from build123d import *

# Parameters (mm, degrees)
EXTRUDE_THIN1_DEPTH     = 60
CUT_EXTRUDE1_DEPTH      = 83.492423895
CUT_EXTRUDE1_DEPTH_BACK = 83.492423895


with BuildPart() as part:
    # Sketch1 → Extrude-Thin1 (new, symmetric)
    with BuildSketch(Plane(origin=(0, 0, 0), x_dir=(1, 0, 0), z_dir=(0, 1, 0))):
        with BuildLine():
            Line((25, -23), (-25, -23))
            ThreePointArc((-25, -23), (-30.656854249, -20.656854249), (-33, -15))
            Line((-33, -15), (-33, 15))
            ThreePointArc((-33, 15), (-30.656854249, 20.656854249), (-25, 23))
            Line((-25, 23), (25, 23))
            ThreePointArc((25, 23), (30.656854249, 20.656854249), (33, 15))
            Line((33, 15), (33, -15))
            ThreePointArc((33, -15), (30.656854249, -20.656854249), (25, -23))
        make_face()
        with BuildLine():
            Line((25, -20), (-25, -20))
            ThreePointArc((-25, -20), (-28.535533906, -18.535533906), (-30, -15))
            Line((-30, -15), (-30, 15))
            ThreePointArc((-30, 15), (-28.535533906, 18.535533906), (-25, 20))
            Line((-25, 20), (25, 20))
            ThreePointArc((25, 20), (28.535533906, 18.535533906), (30, 15))
            Line((30, 15), (30, -15))
            ThreePointArc((30, -15), (28.535533906, -18.535533906), (25, -20))
        make_face(mode=Mode.SUBTRACT)
    extrude(amount=EXTRUDE_THIN1_DEPTH, both=True)

    # Sketch3 → Cut-Extrude1 (cut, two sides: drawn at the far end of the back side and taken through both)
    with BuildSketch(Plane(origin=(0, 0, -23), x_dir=(-1, 0, 0), z_dir=(0, 0, -1)).offset(-CUT_EXTRUDE1_DEPTH_BACK)):
        with BuildLine():
            Line((-5, -40.937612565), (-5, 39.062387435))
            ThreePointArc((-5, 39.062387435), (0, 44.062387435), (5, 39.062387435))
            Line((5, 39.062387435), (5, -40.937612565))
            ThreePointArc((5, -40.937612565), (0, -45.937612565), (-5, -40.937612565))
        make_face()
    extrude(amount=CUT_EXTRUDE1_DEPTH + CUT_EXTRUDE1_DEPTH_BACK, mode=Mode.SUBTRACT)


solid = part.part
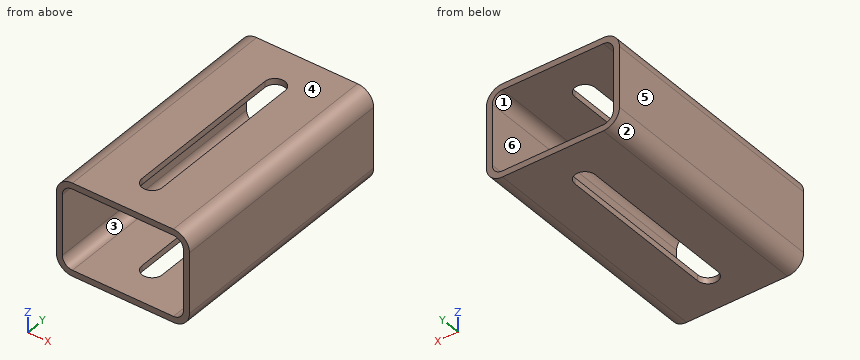
Check sheet for the modelled part. Datum: model origin and axes. Units: mm. Face numbers are marked on the shaded views. A direction names the side the tool comes from. Round coordinates to 2 decimals unless told otherwise and drop trailing zeros. Loops run counter-clockwise (first coordinate to the right, second up) from the corner with the lowest first, then second, coordinate; pieces in that order, holes last. Notation, with made-up numbers: M 71.25,-38.5 L 117.25,-38.5 A28 cw 117.25,-1.5 Z; hole C -19.75,-24 d2. An arc over 180 degrees is marked long. One line per item, written item: value.
(1) Access from +Z, -Z, +X, -X, +Y, -Y to the whole of each face (thin tool, end or side, straight path). Record for the marked faces 5 and 6.
Computed values:
face 5: +Z, -Z, -X, +Y, -Y
face 6: +Y, -Y
(2) Sectioned sample at D-D, the plane x = 0. Record the cut outline in (y, z).
Computed values:
outline: M -60,-23 L -45.94,-23 L -45.94,-20 L -60,-20 Z; M -60,20 L -45.94,20 L -45.94,23 L -60,23 Z; M 44.06,-23 L 60,-23 L 60,-20 L 44.06,-20 Z; M 44.06,20 L 60,20 L 60,23 L 44.06,23 Z
(3) Depth check by flat-ended pin: pin 1 Ø0.9 at (y, z) = (6.5, 22) entering from -X; pin 2 Ø0.9 at (y, z) = (-3.5, -21.5) entering from +X; pin 3 Ø1.5 at (y, z) = (8, -22) entering from -X; pin 4 Ø4 at (x, y) = (-2.5, 21.5) entering from -Z. Enter the tip coordinate at first touch or a pass-through.
Computed values:
pin 1: stops at x = -29.59
pin 2: stops at x = 30.23
pin 3: stops at x = -29.99
pin 4: passes through
(4) Sectioned sample at C-C, the plane x = -17.5. Record the cut outline in (y, z), then the cut area to 3 significant figures.
Computed values:
outline: M -60,-23 L 60,-23 L 60,-20 L -60,-20 Z; M -60,20 L 60,20 L 60,23 L -60,23 Z
area: 720 mm^2
(5) Sectioned sample at B-B, the plane z = 1.5. Record the cut outline in (x, y), then the cut area to 3 significant figures.
Computed values:
outline: M -33,-60 L -30,-60 L -30,60 L -33,60 Z; M 30,-60 L 33,-60 L 33,60 L 30,60 Z
area: 720 mm^2
(6) Release check for a two-part mould opening along Z. For the marked faces 1, 2, 3 and 4 record: +Z half, -Z half, draft (parallel to the pull), parting line (faces both ways), or undercut.
Computed values:
face 1: undercut
face 2: -Z half
face 3: undercut
face 4: +Z half
(7) Sectioned sample at A-A, the plane y = -36.5. Record the cut outline in (x, z), then the cut area to 3 significant figures.
Computed values:
outline: M -33,-15 A8 ccw -25,-23 L -5,-23 L -5,-20 L -25,-20 A5 cw -30,-15 L -30,15 A5 cw -25,20 L -5,20 L -5,23 L -25,23 A8 ccw -33,15 Z; M 5,-23 L 25,-23 A8 ccw 33,-15 L 33,15 A8 ccw 25,23 L 5,23 L 5,20 L 25,20 A5 cw 30,15 L 30,-15 A5 cw 25,-20 L 5,-20 Z
area: 543 mm^2
(8) Thickness scan on line 1 (Z direction, x = 11.5, y = -24); line 2 (X direction, y = -17.5, z = 7); line 3 (Z direction, x = -26, y = 28). Record the ranges inside material, lowest first.
Computed values:
line 1: z = -23 to -20, 20 to 23
line 2: x = -33 to -30, 30 to 33
line 3: z = -22.94 to -19.9, 19.9 to 22.94
